Design review of the part built by this model. Coordinates are the model's own, in mm. A direction names the side the tool comes from. Give positions to 0.01 mm unless a question says otherwise; leave off trailing zeros. Loops run counter-clockwise (first coordinate to the right, second up) from the corner with the lowest first, then second, coordinate; pieces in that order, holes last. Notation, with made-up numbers: M 84.5,-31.75 L 110.5,-31.75 A9 cw 110.5,-24.75 Z; hole C 24.5,28.25 d3. An arc over 180 degrees is marked long. Use a Markdown table: item, result. Add a question column.
(1) Insertion check: pin 1 Ø2 at (x, y) = (21.92, 14) entering from +Z; pin 2 Ø3 at (x, z) = (9.5, 19.5) entering from -Y; pin 3 Ø2 at (x, y) = (21, -14.5) entering from +Z; pin 4 Ø2.5 at (y, z) = (-2, 20) entering from +X. Each pin has a flat end and moves straight along its axis. Give the tip position at first contact, or say it passes through.
(2) Add section A-A, the plane z = 22.5. Give the boundary of the cut face in (x, y).
(3) Add section C-C, the plane x = 15.5. Give the boundary of the cut face in (y, z).
(4) Draft analysis for pull direction Y (two halves, no side actions). For faces 1 (the face through (29.04, 15.61, 20.07)), 2 (the face through (30.465, -17.011, 7.395)), 3 (the face through (21.164, 10.583, 35.07)), state which applies: pulls with the +Y half, pulls with the -Y half, needs draft (parallel to the pull), parting line crosses it, or undercut.
(5) Add section D-D, the plane z = 8.5. Give the boundary of the cut face in (x, y), then the cut area to 3 significant figures.
(6) For faces 4 (the face through (34, 0, 15)), 5 (the face through (22, 12, 30)), 6 (the face through (33.598, 0, 20)), list the 3-axis set-ups (+Z, -Z, +X, -X, +Y, -Y) from which the entire face can be reached by the end or side of a thin tool; tool diameter is ignored.
(7) For probe 1 along Y at (x, z) = (21, 14.5); probe 2 along X at (y, z) = (14, 11); probe 3 along Y at (x, z) = (22, 34.5), list the stretches that pass through material, from the lowest coordinate up.
(8) Add section B-B, the plane y = 0. Give the boundary of the cut face in (x, z).
```python
from build123d import *

# Parameters (mm, degrees)
ESBO_O1_R                = 1.393053459
ESBO_O1_R_2              = 4
RESSALTO_EXTRUS_O1_DEPTH = 40
ESBO_O8_W                = 10
ESBO_O8_H                = 2
ESBO_O10_R               = 3.5
CORTE_EXTRUS_O1_DEPTH    = 10


with BuildPart() as part:
    # Esboço1 → Ressalto-extrusão1 (new body)
    with BuildSketch(Plane.XY):
        with BuildLine():
            Line((0.112562331, -22.423877672), (0.112562331, -19))
            ThreePointArc((0.112562331, -19), (19.112562331, 0), (0.112562331, 19))
            Line((0.112562331, 19), (0.112562331, 22.423877672))
            Line((0.112562331, 22.423877672), (17.598208573, 22.423877672))
            ThreePointArc((17.598208573, 22.423877672), (30.326130634, 17.151799733), (35.598208573, 4.423877672))
            Line((35.598208573, 4.423877672), (35.598208573, -4.423877672))
            ThreePointArc((35.598208573, -4.423877672), (30.326130634, -17.151799733), (17.598208573, -22.423877672))
            Line((17.598208573, -22.423877672), (0.112562331, -22.423877672))
        make_face()
        with Locations((21.9231968, -14)):
            Circle(ESBO_O1_R, mode=Mode.SUBTRACT)
        with Locations((21.9231968, 14)):
            Circle(ESBO_O1_R, mode=Mode.SUBTRACT)
        with Locations((28.9231968, 0)):
            Circle(ESBO_O1_R_2, mode=Mode.SUBTRACT)
    extrude(amount=RESSALTO_EXTRUS_O1_DEPTH)

    # Varredura de corte1: sweep along a path in Esboço9
    with BuildLine(Plane.XY.offset(40)) as varredura_de_corte1_path:
        Line((0.112562331, -22.423877672), (17.598208573, -22.423877672))
        ThreePointArc((17.598208573, -22.423877672), (30.326130634, -17.151799733), (35.598208573, -4.423877672))
        Line((35.598208573, -4.423877672), (35.598208573, 4.423877672))
        ThreePointArc((35.598208573, 4.423877672), (30.326130634, 17.151799733), (17.598208573, 22.423877672))
        Line((17.598208573, 22.423877672), (0.112562331, 22.423877672))
    # Esboço8 → Varredura de corte1 (sweep, cut)
    with BuildSketch(Plane.ZY.offset(-0.112562331)):
        with Locations((20, 21.423877672)):
            Rectangle(ESBO_O8_W, ESBO_O8_H)
    sweep(path=varredura_de_corte1_path.line, mode=Mode.SUBTRACT)

    # Esboço10 → Corte-extrusão1 (cut)
    with BuildSketch(Plane.XY.offset(40)):
        with Locations((21.9231968, 14)):
            Circle(ESBO_O10_R)
        with Locations((21.9231968, -14)):
            Circle(ESBO_O10_R)
    extrude(amount=-CORTE_EXTRUS_O1_DEPTH, mode=Mode.SUBTRACT)


solid = part.part
```
Established:
| question | item | result |
|---|---|---|
| 1 | pin 1 | through |
| 1 | pin 2 | y = -20.42 |
| 1 | pin 3 | z = 30 |
| 1 | pin 4 | x = 33.6 |
| 2 | outline | M 0.11,-20.42 L 17.6,-20.42 A16 ccw 33.6,-4.42 L 33.6,4.42 A16 ccw 17.6,20.42 L 0.11,20.42 L 0.11,19 A19 cw 0.11,-19 Z; hole C 21.92,-14 d2.79; hole C 21.92,14 d2.79; hole C 28.92,0 d8 |
| 3 | outline | M -22.42,0 L -11.15,0 L -11.15,40 L -22.42,40 L -22.42,25 L -20.42,25 L -20.42,15 L -22.42,15 Z; M 11.15,0 L 22.42,0 L 22.42,15 L 20.42,15 L 20.42,25 L 22.42,25 L 22.42,40 L 11.15,40 Z |
| 4 | face 1 | pulls with the +Y half |
| 4 | face 2 | pulls with the -Y half |
| 4 | face 3 | undercut |
| 5 | outline | M 0.11,-22.42 L 17.6,-22.42 A18 ccw 35.6,-4.42 L 35.6,4.42 A18 ccw 17.6,22.42 L 0.11,22.42 L 0.11,19 A19 cw 0.11,-19 Z; hole C 21.92,-14 d2.79; hole C 21.92,14 d2.79; hole C 28.92,0 d8 |
| 5 | area | 823 mm^2 |
| 6 | face 4 | +X |
| 6 | face 5 | +Z |
| 6 | face 6 | +X, +Y, -Y |
| 7 | probe 1 | -22.1 to -15.04, -12.96 to 12.96, 15.04 to 22.1 |
| 7 | probe 2 | 12.96 to 20.53, 23.32 to 32.84 |
| 7 | probe 3 | -21.88 to -17.5, -10.5 to 10.5, 17.5 to 21.88 |
| 8 | outline | M 19.11,0 L 24.92,0 L 24.92,40 L 19.11,40 Z; M 32.92,0 L 35.6,0 L 35.6,15 L 33.6,15 L 33.6,25 L 35.6,25 L 35.6,40 L 32.92,40 Z |
